Design review of the part built by this model. Coordinates are the model's own, in mm. Coordinates: 2 decimals unless noted, no trailing zeros. Order: outer loops, then holes, each group sorted by start corner. A loop starts at its lowest first (then second) coordinate and runs counter-clockwise, first axis right, second up. Notation, with made-up numbers: (19, -15.75) - (59, -15.75) arc R26 cw to (59, 3.25) - close; hole circle Ø6 at (72, 47.5). An arc over 180 degrees is marked (long way). Write item = value, one per line. Start each with the question number.
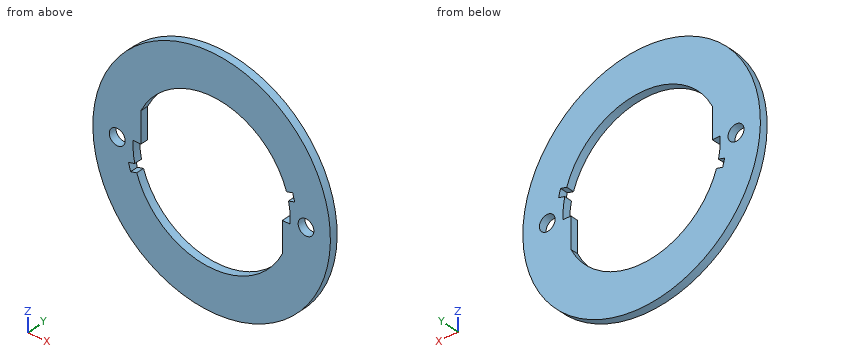
```python
from build123d import *

# Parameters (mm, degrees)
SKETCH1_R           = 47.9425
SKETCH1_R_2         = 3.2131
SKETCH1_R_3         = 3.175
BOSS_EXTRUDE1_DEPTH = 3.175
CUT_EXTRUDE1_DEPTH  = 68.875232873


with BuildPart() as part:
    # Sketch1 → Boss-Extrude1 (new body)
    with BuildSketch(Plane(origin=(0, 0, 0), x_dir=(1, 0, 0), z_dir=(0, 1, 0))):
        with Locations(Location((0, 0, 0), (0, 0, 270))):
            Circle(SKETCH1_R)
        with Locations(Location((-38.1, 0, 0), (0, 0, 270))):
            Circle(SKETCH1_R_2, mode=Mode.SUBTRACT)
        with Locations(Location((38.1, 0, 0), (0, 0, 270))):
            Circle(SKETCH1_R_3, mode=Mode.SUBTRACT)
        with BuildLine():
            Line((-31.710287664, -1.5875), (-28.535287664, -1.5875))
            Line((-28.535287664, -1.5875), (-28.535287664, -13.921201741))
            ThreePointArc((-28.535287664, -13.921201741), (7.915182479, -30.74755903), (31.710287664, 1.5875))
            Line((31.710287664, 1.5875), (28.535287664, 1.5875))
            Line((28.535287664, 1.5875), (28.535287664, 13.921201741))
            ThreePointArc((28.535287664, 13.921201741), (-7.915182479, 30.74755903), (-31.710287664, -1.5875))
        make_face(mode=Mode.SUBTRACT)
    extrude(amount=BOSS_EXTRUDE1_DEPTH)

    # Sketch2 → Cut-Extrude1 (cut, through all)
    with BuildSketch(Plane(origin=(0, 3.175, 0), x_dir=(1, 0, 0), z_dir=(0, 1, 0))):
        Polygon((-33.532471818, 7.341497807), (-32.710721349, 10.408312306), (33.532471818, -7.341497807), (32.710721349, -10.408312306), align=None)
    extrude(amount=-CUT_EXTRUDE1_DEPTH, mode=Mode.SUBTRACT)


solid = part.part
```
Item 1: For P1, Ø1.5, axis at x = -5.5, y = 1, coming from the -Z side; P2, Ø4, axis at x = -38.1, z = 0, coming from the -Y side; P3, Ø1, axis at x = -29.5, y = 1.5, coming from the -Z side; P4, Ø10, axis at x = 38.1, z = 0, coming from the -Y side, all flat-tipped, find the tip position at first contact; note any pin that passes through.
Item 2: Add section B-B on y = 1.1. State how many separate pieces and enclosed holes the cut face has, plus the area to 3 significant figures.
Item 3: Add section D-D on z = -23. Give the boundary of the cut face in (x, y) (1 decimal).
Item 4: For line 1 (X direction, y = 1.1, z = -1.5); line 2 (X direction, y = 0.45, z = -6.5); line 3 (X direction, y = 2.2, z = -4.5), list the stretches that pass through material, from the lowest coordinate up.
Worked out:
q1.P1 = -47.71
q1.P2 = through
q1.P3 = -38.18
q1.P4 = 0
q2.separate_pieces = 1
q2.enclosed_holes = 3
q2.area = 4,020 mm2
q3.outline = (-42.1, 0) - (-21.9, 0) - (-21.9, 3.2) - (-42.1, 3.2) - close; (21.9, 0) - (42.1, 0) - (42.1, 3.2) - (21.9, 3.2) - close
q4.line_1 = -47.92 to -40.94, -35.26 to -31.71, 31.71 to 35.3, 40.9 to 47.92
q4.line_2 = -47.5 to -31.08, 28.54 to 47.5
q4.line_3 = -47.73 to -31.43, 28.54 to 47.73
